Read the model definition and answer for the solid it produces. Units are mm, in the model's axes. A direction names the side the tool comes from. Give positions to 0.01 mm unless a question says otherwise; leave off trailing zeros. Order: outer loops, then holes, each group sorted by start corner. A loop starts at its lowest first (then second) coordinate and runs counter-clockwise, first axis right, second up. Notation, with made-up numbers: (-10, 36) -> (0, 36) arc R8 cw to (0, 44) -> close; hole circle Ø8 at (-12.5, 17.25). An arc over 180 degrees is marked (long way). Answer as CSV lines item,"result". Start each with the question number.
1) Find section C-C (z = 83). Determine the outline of the cut face in (x, y) (3 decimals), and give its area (3 significant figures).
2) Find section B-B (x = 8). Determine the outline of the cut face in (y, z), and give its area (3 significant figures).
3) Straight lines are drawn through the part: L1, parallel to Y at x = 14, z = 86.5; L2, parallel to X at y = -1, z = 104. For each, find the intervals that lie inside material, in ascending order. Write a range as from..to.
4) Find section A-A (y = 2.5). Determine the outline of the cut face in (x, z).
5) For faces 1 (the face through (-0.267, -16.667, 107.463)), 2 (the face through (-16.51, 0, 1)), determine the directions among +Z, -Z, +X, -X, +Y, -Y from which every point of the face is accessible in a straight line to the end or side of a thin tool.
6) The mould has two halves that part along X. Classify faces 3 (the face through (-19.05, 0, 2)), 4 (the face through (0, 16.51, 1)), 5 (the face through (17, 0, -114.3)): +X half, -X half, draft (parallel to the pull), parting line (faces both ways), or undercut.
```python
from build123d import *

# Parameters (mm, degrees)
EXTRUDE_THIN1_DEPTH     = 114.3
CUT_EXTRUDE1_DEPTH      = 1
CUT_EXTRUDE1_DEPTH_BACK = 39.1


with BuildPart() as part:
    # Sketch1 → Extrude-Thin1 (new body, symmetric)
    with BuildSketch(Plane.XY):
        with BuildLine():
            Line((-15.875, 19.05), (15.875, 19.05))
            ThreePointArc((15.875, 19.05), (18.12006403, 18.12006403), (19.05, 15.875))
            Line((19.05, 15.875), (19.05, -15.875))
            ThreePointArc((19.05, -15.875), (18.12006403, -18.12006403), (15.875, -19.05))
            Line((15.875, -19.05), (-15.875, -19.05))
            ThreePointArc((-15.875, -19.05), (-18.12006403, -18.12006403), (-19.05, -15.875))
            Line((-19.05, -15.875), (-19.05, 15.875))
            ThreePointArc((-19.05, 15.875), (-18.12006403, 18.12006403), (-15.875, 19.05))
        make_face()
        with BuildLine():
            Line((-15.875, 16.51), (15.875, 16.51))
            ThreePointArc((15.875, 16.51), (16.324012806, 16.324012806), (16.51, 15.875))
            Line((16.51, 15.875), (16.51, -15.875))
            ThreePointArc((16.51, -15.875), (16.324012806, -16.324012806), (15.875, -16.51))
            Line((15.875, -16.51), (-15.875, -16.51))
            ThreePointArc((-15.875, -16.51), (-16.324012806, -16.324012806), (-16.51, -15.875))
            Line((-16.51, -15.875), (-16.51, 15.875))
            ThreePointArc((-16.51, 15.875), (-16.324012806, 16.324012806), (-15.875, 16.51))
        make_face(mode=Mode.SUBTRACT)
    extrude(amount=EXTRUDE_THIN1_DEPTH, both=True)

    # Sketch3 → Cut-Extrude1 (cut, two sides)
    with BuildSketch(Plane(origin=(0, 19.05, 0), x_dir=(1, 0, 0), z_dir=(0, 1, 0))) as cut_extrude1_sk:
        Polygon((-464.000568463, -276.24876264), (-19.05, -114.3), (19.05, -100.432734074), (464.000568463, 61.516028566), (787.898093744, -828.38510836), (-140.103043182, -1166.149899566), align=None)
    extrude(amount=CUT_EXTRUDE1_DEPTH, mode=Mode.SUBTRACT)
    extrude(cut_extrude1_sk.sketch, amount=-CUT_EXTRUDE1_DEPTH_BACK, mode=Mode.SUBTRACT)


solid = part.part
```
Findings below:
1,outline,"(-19.05, -15.875) arc R3.175 ccw to (-15.875, -19.05) -> (15.875, -19.05) arc R3.175 ccw to (19.05, -15.875) -> (19.05, 15.875) arc R3.175 ccw to (15.875, 19.05) -> (-15.875, 19.05) arc R3.175 ccw to (-19.05, 15.875) -> close; hole (-16.51, -15.875) arc R0.635 ccw to (-15.875, -16.51) -> (15.875, -16.51) arc R0.635 ccw to (16.51, -15.875) -> (16.51, 15.875) arc R0.635 ccw to (15.875, 16.51) -> (-15.875, 16.51) arc R0.635 ccw to (-16.51, 15.875) -> close"
1,area,"353 mm²"
2,outline,"(-19.05, -114.3) -> (-16.51, -114.3) -> (-16.51, 104.45) -> (-19.05, 104.45) -> close; (16.51, -114.3) -> (19.05, -114.3) -> (19.05, 104.45) -> (16.51, 104.45) -> close"
2,area,"1,110 mm²"
3,L1,"-19.05..-16.51, 16.51..19.05"
3,L2,"-19.05..-16.51"
4,outline,"(-19.05, -114.3) -> (-16.51, -114.3) -> (-16.51, 113.38) -> (-19.05, 114.3) -> close; (16.51, -114.3) -> (19.05, -114.3) -> (19.05, 100.43) -> (16.51, 101.36) -> close"
5,face 1,"+Z, +X, +Y, -Y"
5,face 2,"+Z, -Z"
6,face 3,"-X half"
6,face 4,"undercut"
6,face 5,"draft"
